from build123d import *

# Parameters (mm, degrees)
CYLINDER_R      = 2.5
CYLINDER_DEPTH  = 8.5
TUBE_R          = 5
TUBE_R_2        = 3.55
TUBE_DEPTH      = 2.5
EXTRUDE_DEPTH   = 8.5
CHAMFER_SIZE    = 0.2
CHAMFER001_SIZE = 0.4


with BuildPart() as cylindre:
    # Cylinder → Cylinder (new body)
    with BuildSketch(Plane(origin=(0, 0.79, 0), x_dir=(1, 0, 0), z_dir=(0, 0, 1))):
        Circle(CYLINDER_R)
    extrude(amount=CYLINDER_DEPTH)


with BuildPart() as tube:
    # Tube → Tube (new body)
    with BuildSketch(Plane.XY):
        Circle(TUBE_R)
        Circle(TUBE_R_2, mode=Mode.SUBTRACT)
    extrude(amount=TUBE_DEPTH)


with BuildPart() as chamfer001:
    # RegularPolygon → Extrude (new body)
    with BuildSketch(Plane(origin=(0, 0, 0), x_dir=(0, 1, 0), z_dir=(0, 0, 1))):
        Polygon((0, -5), (4.330127, -2.5), (4.330127, 2.5), (0, 5), (-4.330127, 2.5), (-4.330127, -2.5), align=None)
    extrude(amount=EXTRUDE_DEPTH)

    # Cut: cut Tube
    add(tube.part, mode=Mode.SUBTRACT)

    # Cut001: cut Cylindre
    add(cylindre.part, mode=Mode.SUBTRACT)

    # Chamfer
    chamfer_edges = [chamfer001.edges().sort_by_distance(p)[0] for p in [
        (2.5, 4.330127, 5.5),
        (5, 0, 5.5),
        (-2.5, 4.330127, 5.5),
        (2.5, -4.330127, 5.5),
        (-2.5, -4.330127, 5.5),
        (-5, 0, 5.5),
    ]]
    chamfer(chamfer_edges, length=CHAMFER_SIZE)

    # Chamfer001
    chamfer001_edges = [chamfer001.edges().sort_by_distance(p)[0] for p in [
        (4.9, 0, 2.5),
        (2.45, 4.243524, 2.5),
        (-2.45, 4.243524, 2.5),
        (-4.9, 0, 2.5),
        (-2.45, -4.243524, 2.5),
        (2.45, -4.243524, 2.5),
        (4.9, 0, 8.5),
        (2.45, 4.243524, 8.5),
        (-2.45, 4.243524, 8.5),
        (-4.9, 0, 8.5),
        (-2.45, -4.243524, 8.5),
        (2.45, -4.243524, 8.5),
    ]]
    chamfer(chamfer001_edges, length=CHAMFER001_SIZE)


solid = chamfer001.part
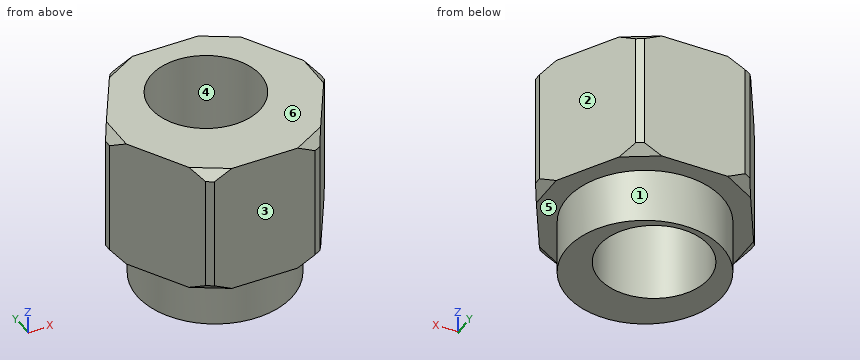
Verification items for the finished model (mm, model axes). Face numbers are marked on the shaded views. A direction names the side the tool comes from. Coordinates: 2 decimals unless noted, no trailing zeros. Write each loop counter-clockwise with the first axis right and the second up, starting at its lowest first coordinate (ties: lowest second). Pieces come first, ordered by that corner, then holes. Notation, with made-up numbers: (20, 54) -> (51, 54) arc R9 ccw to (51, 65) -> close; hole circle Ø9 at (44.5, 3). An arc over 180 degrees is marked (long way). One line per item, written item: value. Start each with the question number.
Q1. Access from +Z, -Z, +X, -X, +Y, -Y to the whole of each face (thin tool, end or side, straight path). Record for the marked faces 5 and 6.
Q2. Cross-section at A-A on x = 0. Enter the section's corners in (y, z).
Q3. Cross-section at D-D on x = -1.25. Enter the section's corners in (y, z).
Q4. Cross-section at C-C on z = 2. Enter the section's corners in (x, y), and give its area (3 significant figures).
Q5. Mould release check, pull along X, two halves, no side actions. Record for the marked faces 1, 2, 3 and 4: pulls with the +X half, pulls with the -X half, needs draft (parallel to the pull), parting line crosses it, or undercut.
Q6. Thickness scan on L1, parallel to Y at x = 0, z = 3.5; L2, parallel to Y at x = 0, z = 1.5; L3, parallel to Z at x = 1.75, y = -3.25. Record the ranges inside material, lowest first. Write a range as from..to.
Q7. Cross-section at B-B on y = 0. Enter the section's corners in (x, z).
Q8. Go/stop test with flat-tipped pins: P1, Ø3, axis at x = -4, z = 2.5, coming from the -Y side; P2, Ø1, axis at x = -3.5, y = 2.5, coming from the -Z side; P3, Ø3, axis at y = -2, z = 2, coming from the +X side. Record where each tip stops, or that it passes through.
Checked values:
1. face 5: -Z
1. face 6: +Z, +X, -X, +Y, -Y
2. outline: (-4.33, 2.5) -> (-3.55, 2.5) -> (-3.55, 0) -> (-1.71, 0) -> (-1.71, 8.5) -> (-4.33, 8.5) -> close; (3.29, 0) -> (3.55, 0) -> (3.55, 2.5) -> (4.33, 2.5) -> (4.33, 8.5) -> (3.29, 8.5) -> close
3. outline: (-4.33, 2.5) -> (-3.32, 2.5) -> (-3.32, 0) -> (-1.38, 0) -> (-1.38, 8.5) -> (-4.33, 8.5) -> close; (2.96, 0) -> (3.32, 0) -> (3.32, 2.5) -> (4.33, 2.5) -> (4.33, 8.5) -> (2.96, 8.5) -> close
4. outline: circle Ø7.1 at (0, 0); hole circle Ø5 at (0, 0.79)
4. area: 20.0 mm²
5. face 1: parting line crosses it
5. face 2: pulls with the +X half
5. face 3: needs draft
5. face 4: undercut
6. L1: y = -4.33..-1.71, 3.29..4.33
6. L2: y = -3.55..-1.71, 3.29..3.55
6. L3: z = 2.5..8.5
7. outline: (-4.9, 2.9) -> (-4.5, 2.5) -> (-3.55, 2.5) -> (-3.55, 0) -> (-2.37, 0) -> (-2.37, 8.5) -> (-4.5, 8.5) -> (-4.9, 8.1) -> close; (2.37, 0) -> (3.55, 0) -> (3.55, 2.5) -> (4.5, 2.5) -> (4.9, 2.9) -> (4.9, 8.1) -> (4.5, 8.5) -> (2.37, 8.5) -> close
8. P1: stops at y = -4.18
8. P2: stops at z = 2.5
8. P3: stops at x = 4.63
